Read the model definition and answer for the solid it produces. Units are mm, in the model's axes. Coordinates: 2 decimals unless noted, no trailing zeros. Order: outer loops, then holes, each group sorted by start corner. A loop starts at its lowest first (then second) coordinate and runs counter-clockwise, first axis right, second up. Notation, with made-up numbers: (-19.75, -10) - (20.25, -10) arc R20 ccw to (20.25, 24) - close; hole circle Ø5 at (44.5, 59). An arc over 180 degrees is marked (long way). Answer as a JSON object with one key per item and string values. Group by question number.
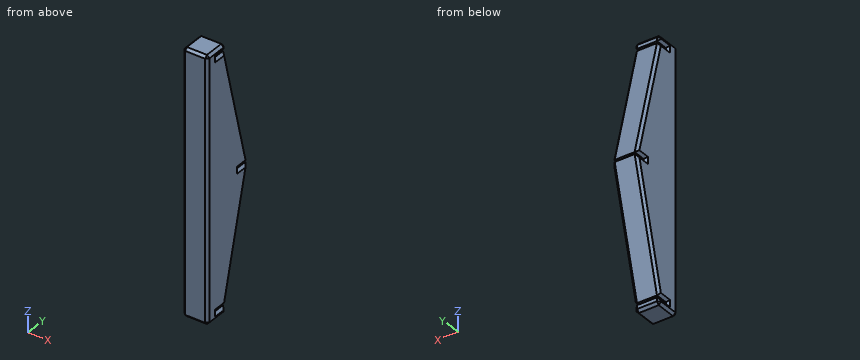
from build123d import *

# Parameters (mm, degrees)
PAD005_DEPTH            = 20
CHAMFER_SIZE            = 2
BODY003_ROLL_ANGLE      = 90
BODY003_PLACEMENT_ANGLE = 90


with BuildPart() as sideholder1:
    # Sketch006 → Pad005 (new body)
    with BuildSketch(Plane.XY):
        Polygon((0, -105), (20, -105), (20, -100), (10, -100), (10, -98.4), (20, -98.4), (45, -1.6), (35, -1.6), (35, 0), (45, 0), (20, 98.4), (10, 98.4), (10, 100), (20, 100), (20, 105), (0, 105), align=None)
    extrude(amount=PAD005_DEPTH)

    # Chamfer
    chamfer_edges = [sideholder1.edges().sort_by_distance(p)[0] for p in [
        (10, -105, 20),
        (20, -102.5, 20),
        (15, -100, 20),
        (10, -99.2, 20),
        (15, -98.4, 20),
        (32.5, -50, 20),
        (40, -1.6, 20),
        (35, -0.8, 20),
        (40, 0, 20),
        (32.5, 49.2, 20),
        (15, 98.4, 20),
        (10, 99.2, 20),
        (15, 100, 20),
        (20, 102.5, 20),
        (10, 105, 20),
        (0, 0, 20),
        (10, -105, 0),
        (20, -102.5, 0),
        (15, -100, 0),
        (10, -99.2, 0),
        (15, -98.4, 0),
        (32.5, -50, 0),
        (40, -1.6, 0),
        (35, -0.8, 0),
        (40, 0, 0),
        (32.5, 49.2, 0),
        (15, 98.4, 0),
        (10, 99.2, 0),
        (15, 100, 0),
        (20, 102.5, 0),
        (10, 105, 0),
        (0, 0, 0),
        (0, 105, 10),
        (0, -105, 10),
        (20, 105, 10),
        (20, -105, 10),
    ]]
    chamfer(chamfer_edges, length=CHAMFER_SIZE)


with BuildPart() as sideholder1_1:
    # Body003 roll: moved
    add(sideholder1.part.rotate(Axis((0, 0, 0), (1, 0, 0)), BODY003_ROLL_ANGLE))


with BuildPart() as sideholder1_2:
    # Body003 placement: moved
    add(sideholder1_1.part.moved(Location((120, -185, 0))).rotate(Axis((120, -185, 0), (0, 0, 1)), BODY003_PLACEMENT_ANGLE))


with BuildPart() as sideholder2_mirror:
    # mirror: instance of SideHolder1
    add(sideholder1_2.part.mirror(Plane(origin=(0, 0, 0), x_dir=(0, -1, 0), z_dir=(1, 0, 0))))


solid = sideholder2_mirror.part
1. Straight lines are drawn through the part: L1, parallel to Z at x = -137.75, y = -167; L2, parallel to Z at x = -138.5, y = -173; L3, parallel to Y at x = -129.25, z = 92. For each, find the intervals that lie inside material, in ascending order.
2. Given pin 1 (10 mm diameter, centred on x = -137, z = 78, fed in from +Y); pin 2 (0.5 mm diameter, centred on x = -131.5, z = 99, fed in from +Y); pin 3 (6 mm diameter, centred on x = -127.5, z = -21.5, fed in from +Y), each flat-ended and moving along its own axis, determine where each tip first touches the part or whether it passes through.
3. A cutting plane is placed at B-B on z = -38.5. Write down the section's boundary in (x, y).
4. A cutting plane is placed at A-A on x = -129. Write down the section's boundary in (y, z), and give its area (3 significant figures).
5. A cutting plane is placed at C-C on y = -162. Write down the section's boundary in (x, z).
Derived:
{
 "1": {"L1": "z = -105 to -100, -98.4 to 98.4, 100 to 105", "L2": "z = -104.5 to -100.5, -97.9 to 97.9, 100.5 to 104.5", "L3": "y = -185 to -163.37"},
 "2": {"pin 1": "stops at y = -158.55", "pin 2": "stops at y = -175", "pin 3": "stops at y = -144.36"},
 "3": {"outline": "(-140, -183) - (-138, -185) - (-122, -185) - (-120, -183) - (-120, -151.6) - (-122, -149.53) - (-138, -149.53) - (-140, -151.6) - close"},
 "4": {"outline": "(-185, -103) - (-183, -105) - (-167, -105) - (-165, -103) - (-165, -100) - (-175, -100) - (-175, -98.4) - (-165, -98.4) - (-140, -1.6) - (-150, -1.6) - (-150, 0) - (-140, 0) - (-165, 98.4) - (-175, 98.4) - (-175, 100) - (-165, 100) - (-165, 103) - (-167, 105) - (-183, 105) - (-185, 103) - close", "area": "6,620 mm2"},
 "5": {"outline": "(-140, -78.79) - (-138, -86.78) - (-122, -86.78) - (-120, -78.79) - (-120, 78.47) - (-122, 86.59) - (-138, 86.59) - (-140, 78.47) - close"}
}
